Read the model definition and answer for the solid it produces. Units are mm, in the model's axes. A direction names the side the tool comes from. Coordinates: 2 decimals unless noted, no trailing zeros. Write each loop counter-clockwise with the first axis right and the second up, starting at its lowest first coordinate (ties: lowest second). Pieces come first, ordered by that corner, then holes.
(1) Section C-C on x = 0 is taken. Write down the section's boundary in (y, z), then the cut area to 3 significant figures.
(2) Section D-D on z = 2 is taken. Write down the section's boundary in (x, y), then the cut area to 3 significant figures.
(3) Section A-A on y = 0 is taken. Write down the section's boundary in (x, z).
(4) Find the intervals of material crossed by probe 1 along Y at (x, z) = (0, 10.75); probe 2 along X at (y, z) = (0.5, 14); probe 3 along Z at (x, y) = (-7, 7.5), in increasing order.
(5) The mould has two halves that part along Y. Classify faces 3 (the conical face through (19.166, 6.036, 0.194)), 4 (the flat face through (0, 0, 0)), 5 (the cylindrical face through (-10, 0, 2)): +Y half, -Y half, draft (parallel to the pull), parting line (faces both ways), or undercut.
(6) Which of the six approach directions +Z, -Z, +X, -X, +Y, -Y give full straight-line access (tool end or side, diameter ignored) to faces 1 (the flat face through (1.7, -21.1, 24)), 2 (the flat face through (0, 0, 5))?
(7) Section B-B on z = 14.25 is taken. Write down the section's boundary in (x, y), then the cut area to 3 significant figures.
(8) Given pin 1 (5 mm diameter, centred on x = -8, z = 5, fed in from -Y); pin 2 (8 mm diameter, centred on y = 6.5, z = 20.5, fed in from -X); pin 3 (1.5 mm diameter, centred on x = -14.5, z = 7.5, fed in from +Y), each flat-ended and moving along its own axis, determine where each tip first touches the part or whether it passes through.
from build123d import *

# Parameters (mm, degrees)
F2_SIZE = 2
F3_SIZE = 4
F5_D    = 5


with BuildPart() as f1:
    # F0 (on Front) → F1 (revolve)
    with BuildSketch(Plane.XZ):
        Polygon((0, 5), (0, 0), (23.9, 0), (23.9, 24), (19, 24), (19, 5), align=None)
    revolve(axis=Axis((0, 0, 12.3709159863), (0, 0, 1)))

    # F2
    f2_edges = [f1.edges().sort_by_distance(p)[0] for p in [
        (-19, 0, 24),
    ]]
    chamfer(f2_edges, length=F2_SIZE)

    # F3
    f3_edges = [f1.edges().sort_by_distance(p)[0] for p in [
        (-23.9, 0, 0),
    ]]
    chamfer(f3_edges, length=F3_SIZE)

    # F5 (through all)
    with Locations(Plane.XY.offset(5)):
        with Locations((-12.5, 0), (12.5, 0)):
            Hole(F5_D / 2)


solid = f1.part
Response:
1. outline: (-23.9, 4) - (-19.9, 0) - (19.9, 0) - (23.9, 4) - (23.9, 24) - (21, 24) - (19, 22) - (19, 5) - (-19, 5) - (-19, 22) - (-21, 24) - (-23.9, 24) - close
1. area: 405 mm2
2. outline: circle Ø43.8 at (0, 0); hole circle Ø5 at (-12.5, 0); hole circle Ø5 at (12.5, 0)
2. area: 1,470 mm2
3. outline: (-23.9, 4) - (-19.9, 0) - (-15, 0) - (-15, 5) - (-19, 5) - (-19, 22) - (-21, 24) - (-23.9, 24) - close; (-10, 0) - (10, 0) - (10, 5) - (-10, 5) - close; (15, 0) - (19.9, 0) - (23.9, 4) - (23.9, 24) - (21, 24) - (19, 22) - (19, 5) - (15, 5) - close
4. probe 1: y = -23.9 to -19, 19 to 23.9
4. probe 2: x = -23.89 to -18.99, 18.99 to 23.89
4. probe 3: z = 0 to 5
5. face 3: parting line
5. face 4: draft
5. face 5: undercut
6. face 1: +Z, +X, -X, +Y, -Y
6. face 2: +Z
7. outline: circle Ø47.8 at (0, 0); hole circle Ø38 at (0, 0)
7. area: 660 mm2
8. pin 1: stops at y = -23.26
8. pin 2: stops at x = -23.77
8. pin 3: stops at y = 19.55
